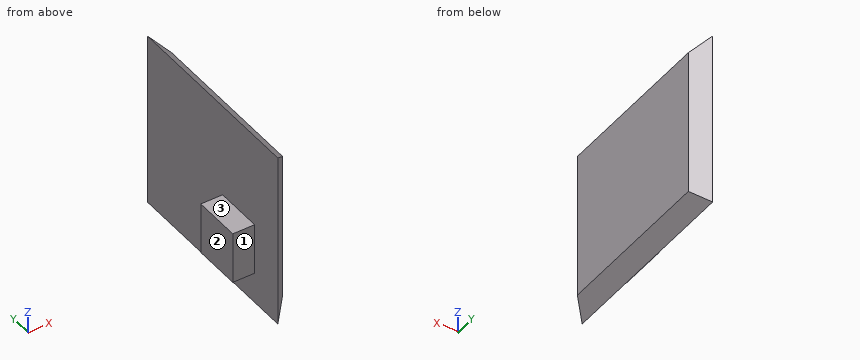
from build123d import *

# Parameters (mm, degrees)
F0_W     = 114.0731200576
F0_H     = 101.4817282557
F1_DEPTH = 10
F1_TAPER = -45
F2_W     = 32.8839123249
F2_H     = 35.4949785396
F3_DEPTH = 25


with BuildPart() as f1:
    # F0 (on Right) → F1 (new body)
    with BuildSketch(Plane.YZ):
        with Locations((23.8430835307, 1.4738403261)):
            Rectangle(F0_W, F0_H)
    extrude(amount=-F1_DEPTH, taper=F1_TAPER)

    # F2 (on face) → F3 (join)
    with BuildSketch(Plane.YZ):
        with Locations((-2.8988905251, -20.2437178232)):
            Rectangle(F2_W, F2_H)
    extrude(amount=-F3_DEPTH)


solid = f1.part
Build history of the part. All positions in model axes, mm. Face numbers are marked on the shaded views. A direction names the side the tool comes from. Give positions to 0.01 mm unless a question says otherwise; leave off trailing zeros. Order: outer loops, then holes, each group sorted by start corner. A loop starts at its lowest first (then second) coordinate and runs counter-clockwise, first axis right, second up. Notation, with made-up numbers: M 55,86 L 65,86 A13 cw 65,109 Z; hole C 21,52 d6. An arc over 180 degrees is marked long. Use one line per item in the form item = value.
1) Tool access for the marked faces 1, 2 and 3: list every direction of +Z, -Z, +X, -X, +Y, -Y with a clear straight run to the whole face (end or side of a thin tool).
Calculated:
face_1 = +Z, -Z, -X, -Y
face_2 = +Z, -Z, -X, +Y, -Y
face_3 = +Z, -X, +Y, -Y
2) Drop flat-ended pins along their axis: pin 1 (1.5 mm diameter, centred on y = 2.5, z = 0.5, fed in from -X); pin 2 (1.5 mm diameter, centred on x = -8, z = 0.5, fed in from -Y); pin 3 (12 mm diameter, centred on x = -15, z = -7, fed in from -Y). Give the stop position or say it passes through.
Calculated:
pin_1 = -10
pin_2 = -41.94
pin_3 = -43.19
3) Saw through at A-A (x = -21.5). Give the cut face in (y, z), plus the area to 3 significant figures.
Calculated:
outline = M -19.34,-37.99 L 13.54,-37.99 L 13.54,-2.5 L -19.34,-2.5 Z
area = 1,170 mm2
4) Probe probe 1 along X at (y, z) = (38, -6.5); probe 2 along Z at (x, y) = (-10.5, 12); probe 3 along Y at (x, z) = (-19.5, -32). List the from-to ranges inside material, lowest first.
Calculated:
probe_1 = -10 to 0
probe_2 = -37.99 to -2.5
probe_3 = -19.34 to 13.54
